Could you check a few things on this model? Use its own coordinates, in mm. Round coordinates to 2 decimals unless told otherwise and drop trailing zeros.
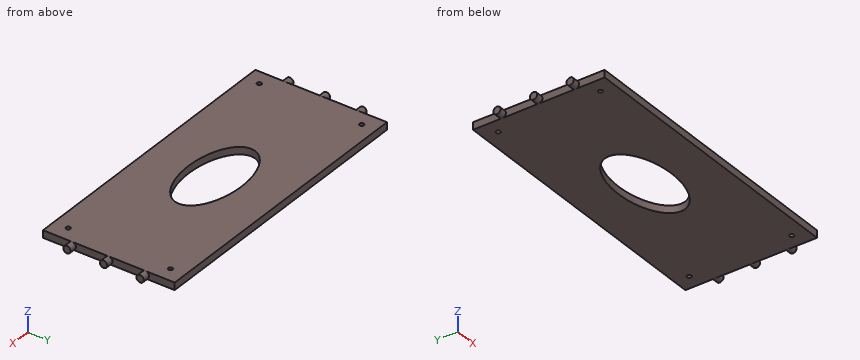
from build123d import *

# Parameters (mm, degrees)
SKETCH1_W           = 200
SKETCH1_H           = 90
BOSS_EXTRUDE1_DEPTH = 5
SKETCH2_R           = 2.5
BOSS_EXTRUDE2_DEPTH = 5
SKETCH3_R           = 1.5
SKETCH3_RX          = 34.171351791
SKETCH3_RY          = 17.990877267
CUT_EXTRUDE1_DEPTH  = 5


with BuildPart() as part:
    # Sketch1 → Boss-Extrude1 (new body)
    with BuildSketch(Plane.XY):
        Rectangle(SKETCH1_W, SKETCH1_H)
    extrude(amount=BOSS_EXTRUDE1_DEPTH)

    # Sketch2 → Boss-Extrude2 (add)
    with BuildSketch(Plane(origin=(100, 0, 0), x_dir=(0, 0, -1), z_dir=(1, 0, 0))):
        with Locations((-2.5, 25)):
            Circle(SKETCH2_R)
        with Locations((-2.5, 0)):
            Circle(SKETCH2_R)
        with Locations((-2.5, -25)):
            Circle(SKETCH2_R)
    boss_extrude2 = extrude(amount=BOSS_EXTRUDE2_DEPTH)

    # Mirror1: Boss-Extrude2 across plane
    add(boss_extrude2.mirror(Plane(origin=(0, 0, 0), x_dir=(0, 0, 1), z_dir=(1, 0, 0))))

    # Sketch3 → Cut-Extrude1 (cut)
    with BuildSketch(Plane(origin=(0, 0, 0), x_dir=(-1, 0, 0), z_dir=(0, 0, -1))):
        with Locations((-90, 35)):
            Circle(SKETCH3_R)
        with Locations(Location((-90, -35, 0), (0, 0, 180))):
            Circle(SKETCH3_R)
        with Locations((90, -35)):
            Circle(SKETCH3_R)
        with Locations(Location((90, 35, 0), (0, 0, 180))):
            Circle(SKETCH3_R)
        with Locations((0, 0)):
            Ellipse(SKETCH3_RX, SKETCH3_RY)
    extrude(amount=-CUT_EXTRUDE1_DEPTH, mode=Mode.SUBTRACT)


solid = part.part
Item 1: Will these pins go through, and if not, where does the flat tip stop? pin 1 (1.5 mm diameter, centred on y = 35, z = 2.5, fed in from -X); pin 2 (2.5 mm diameter, centred on x = -90, y = -35, fed in from -Z); pin 3 (2.5 mm diameter, centred on y = -7, z = 3.5, fed in from +X).
Results list:
pin 1: stops at x = -100
pin 2: passes through
pin 3: stops at x = 100
Item 2: If we section it at A-A, the plane z = 2: Count the separate pieces of the cut face and the enclosed holes in it, then the cut area to 3 significant figures.
Results list:
separate pieces: 1
enclosed holes: 5
area: 16,200 mm2
Item 3: If I drill on line 1 along Y through (x, z) = (90, 1.25); line 2 along X through (y, z) = (-31.5, 1.6); line 3 along X through (y, z) = (-2.5, 1.55), over which ranges is the centre line in solid material (lowest first)?
Results list:
line 1: y = -45 to -36.5, -33.5 to 33.5, 36.5 to 45
line 2: x = -100 to 100
line 3: x = -100 to -33.84, 33.84 to 100
